```python
from build123d import *

# Parameters (mm, degrees)
SKETCH_1_R               = 15
SKETCH_1_R_2             = 4
EXTRUDE_1_DEPTH          = 3
SKETCH_2_R               = 7
SKETCH_2_R_2             = 4
EXTRUDE_2_DEPTH          = 7
CUT_EXTRUDE_1_DEPTH      = 13
CUT_EXTRUDE_1_DEPTH_BACK = 12
SKETCH_5_R               = 1.5
SKETCH_7_R               = 1.5
CUT_EXTRUDE_3_DEPTH      = 4
CHAMFER_1_SIZE           = 1


with BuildPart() as part:
    # Sketch 1 → Extrude 1 (new body)
    with BuildSketch(Plane(origin=(0, 0, 0), x_dir=(1, 0, 0), z_dir=(0, 1, 0))):
        with Locations(Location((0, 0, 0), (0, 0, 270))):
            Circle(SKETCH_1_R)
        with Locations(Location((0, 0, 0), (0, 0, 270))):
            Circle(SKETCH_1_R_2, mode=Mode.SUBTRACT)
    extrude(amount=EXTRUDE_1_DEPTH)

    # Sketch 2 → Extrude 2 (add)
    with BuildSketch(Plane(origin=(0, 3, 0), x_dir=(1, 0, 0), z_dir=(0, 1, 0))):
        with Locations(Location((0, 0, 0), (0, 0, 270))):
            Circle(SKETCH_2_R)
        with Locations(Location((0, 0, 0), (0, 0, 270))):
            Circle(SKETCH_2_R_2, mode=Mode.SUBTRACT)
    extrude(amount=EXTRUDE_2_DEPTH)

    # Sketch 5 → Cut-Extrude 1 (cut, two sides: drawn at the far end of the back side and taken through both)
    with BuildSketch(Plane.ZY.offset(-CUT_EXTRUDE_1_DEPTH_BACK)):
        with Locations((0, 5.8)):
            Circle(SKETCH_5_R)
    extrude(amount=CUT_EXTRUDE_1_DEPTH + CUT_EXTRUDE_1_DEPTH_BACK, mode=Mode.SUBTRACT)

    # Sketch 7 → Cut-Extrude 3 (cut)
    with BuildSketch(Plane(origin=(0, 3, 0), x_dir=(1, 0, 0), z_dir=(0, 1, 0))):
        with Locations(Location((12, 0, 0), (0, 0, 270))):
            Circle(SKETCH_7_R)
        with Locations(Location((0, -12, 0), (0, 0, 270))):
            Circle(SKETCH_7_R)
        with Locations(Location((-12, 0, 0), (0, 0, 270))):
            Circle(SKETCH_7_R)
        with Locations(Location((0, 12, 0), (0, 0, 270))):
            Circle(SKETCH_7_R)
    extrude(amount=-CUT_EXTRUDE_3_DEPTH, mode=Mode.SUBTRACT)

    # Chamfer 1
    chamfer_1_edges = [part.edges().sort_by_distance(p)[0] for p in [
        (0, 10, -4),
    ]]
    chamfer(chamfer_1_edges, length=CHAMFER_1_SIZE)


solid = part.part
```
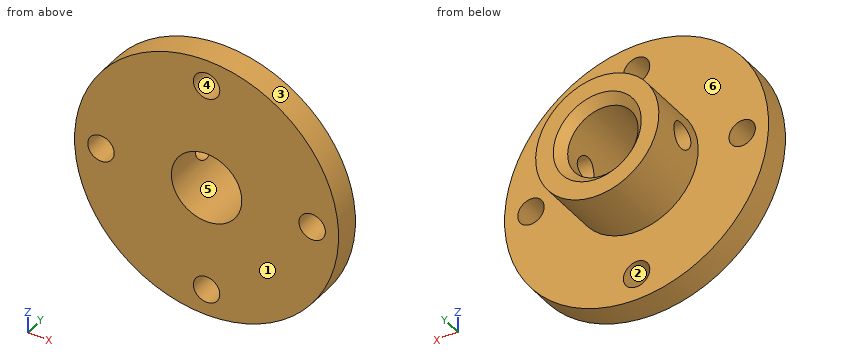
Geometry check sheet. Reference: the model listing, model coordinates, mm. Face numbers are marked on the shaded views. A direction names the side the tool comes from. Round coordinates to 2 decimals unless told otherwise and drop trailing zeros. Order: outer loops, then holes, each group sorted by start corner. A loop starts at its lowest first (then second) coordinate and runs counter-clockwise, first axis right, second up. Notation, with made-up numbers: (82.5, 22) -> (125.5, 22) arc R6 cw to (125.5, 27) -> close; hole circle Ø5 at (43.5, 39.5). An arc over 180 degrees is marked (long way). Return JSON: item names as keys, results as strings. Group by question number.
Q1. Section check D-D, the plane z = -0.25. Count the separate pieces of the cut face and the enclosed holes in it, plus the area to 3 significant figures.
Q2. Section check A-A, the plane x = -12. Record the boundary of the cut face in (y, z).
Q3. Material ranges on probe 1 along X at (y, z) = (2.2, 0); probe 2 along X at (y, z) = (3.25, 0); probe 3 along Y at (x, z) = (5, -5.5), recorded low to high. Write a range as from..to.
Q4. Gauge pin test, flat ends, axial feed: pin 1 (2.5 mm diameter, centred on y = 5.8, z = 0, fed in from -X); pin 2 (1 mm diameter, centred on y = 3, z = -5, fed in from +X); pin 3 (5 mm diameter, centred on y = 5.8, z = 0, fed in from +X); pin 4 (5 mm diameter, centred on x = -11, z = 7.5, fed in from +Y). Record the tip position at first contact, or that the pin passes through.
Q5. Release check for a two-part mould opening along Z. For the marked faces 1, 2, 3 and 4 record: released by +Z, released by -Z, zero draft, split by the parting line, or undercut.
Q6. Section check C-C, the plane x = 0. Record the boundary of the cut face in (y, z), plus the area to 3 significant figures.
Q7. Tool access check on the marked faces 5 and 6. Record the directions out of +Z, -Z, +X, -X, +Y, -Y that give a thin tool (end or side, any length) a straight path to the whole face; none if there is none.
Q8. Section check B-B, the plane z = -12. Record the boundary of the cut face in (x, y).
Numbers:
{
 "1": {"separate pieces": "6", "enclosed holes": "0", "area": "71.6 mm^2"},
 "2": {"outline": "(0, -9) -> (3, -9) -> (3, -1.5) -> (0, -1.5) -> close; (0, 1.5) -> (3, 1.5) -> (3, 9) -> (0, 9) -> close"},
 "3": {"probe 1": "-15..-13.5, -10.5..-4, 4..10.5, 13.5..15", "probe 2": "-7..-4, 4..7", "probe 3": "0..3"},
 "4": {"pin 1": "through", "pin 2": "x = 14.31", "pin 3": "x = 7", "pin 4": "y = 3"},
 "5": {"face 1": "zero draft", "face 2": "undercut", "face 3": "split by the parting line", "face 4": "undercut"},
 "6": {"outline": "(0, -15) -> (3, -15) -> (3, -13.5) -> (0, -13.5) -> close; (0, -10.5) -> (3, -10.5) -> (3, -7) -> (10, -7) -> (10, -5) -> (9, -4) -> (0, -4) -> close; (0, 4) -> (9, 4) -> (10, 5) -> (10, 7) -> (3, 7) -> (3, 10.5) -> (0, 10.5) -> close; (0, 13.5) -> (3, 13.5) -> (3, 15) -> (0, 15) -> close", "area": "89.0 mm^2"},
 "7": {"face 5": "+Y, -Y", "face 6": "+Y"},
 "8": {"outline": "(-9, 0) -> (-1.5, 0) -> (-1.5, 3) -> (-9, 3) -> close; (1.5, 0) -> (9, 0) -> (9, 3) -> (1.5, 3) -> close"}
}
